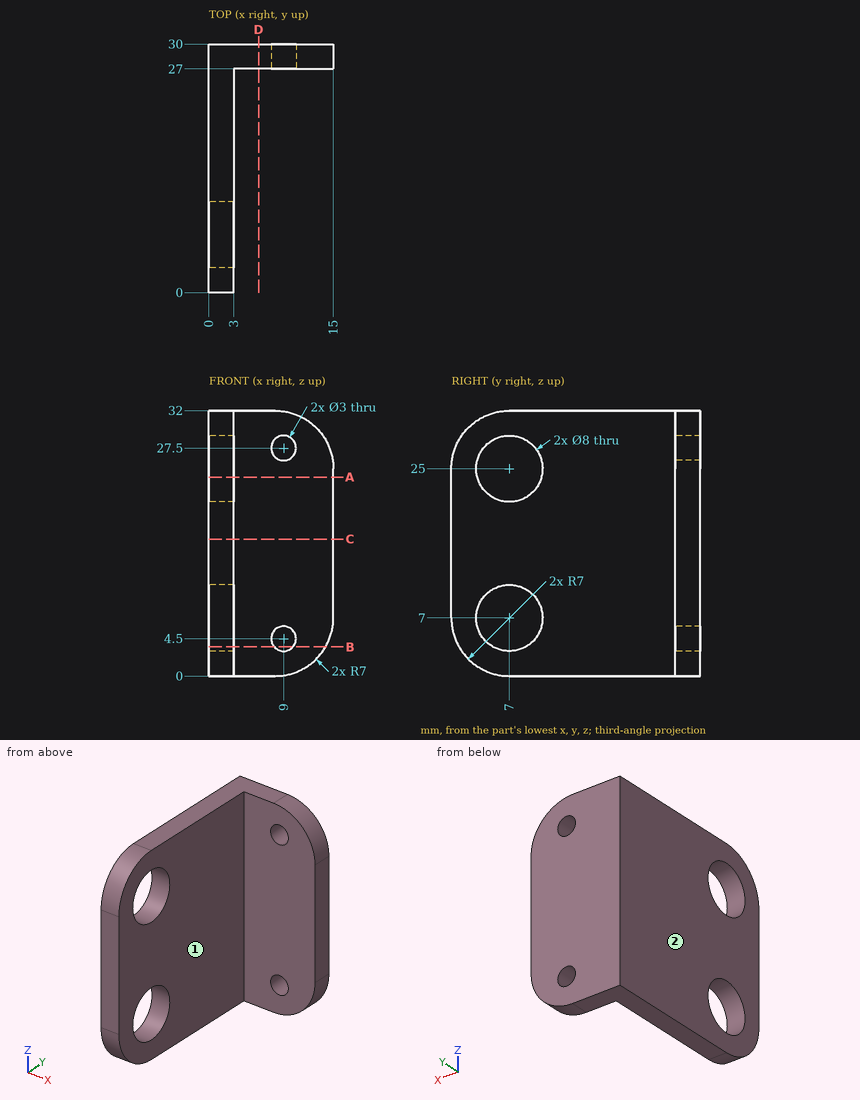
Input: dimensioned drawing with shaded views. Units: mm. Origin: part minimum x, y, z. A direction names the side the tool comes from. Give positions to 0.01 mm unless a question says otherwise; leave off trailing zeros. Loops run counter-clockwise (first coordinate to the right, second up) from the corner with the lowest first, then second, coordinate; pieces in that order, holes last. Notation, with made-up numbers: (16, 76) -> (28, 76) arc R21 cw to (28, 109) -> close; hole circle Ø3 at (-28.5, 77.5). An arc over 180 degrees is marked (long way). Use a Markdown table: item, result. Add a question column.
1) Section query C-C, the plane z = 16.5. Return the cut outline in (x, y), then the cut area to 3 significant figures.
2) Section query A-A, the plane z = 24. Return the cut outline in (x, y), then the cut area to 3 significant figures.
3) Section query B-B, the plane z = 3.5. Return the cut outline in (x, y).
4) Line query: line 1 along Z through (x, y) = (1.1, 7); line 2 along Z through (x, y) = (2.75, 4); line 3 along Y through (x, z) = (1.25, 25). Output: solid intervals per line, ascending. Write a range as [from, to].
5) Section query D-D, the plane x = 6. Return the cut outline in (y, z), then the cut area to 3 significant figures.
6) Reachability of the marked faces 1 and 2 from +Z, -Z, +X, -X, +Y, -Y: full face, straight path, thin tool, end or side. Return the list, or none.
7) First-contact query: pin 1 (5 mm diameter, centred on y = 19.5, z = 27.5, fed in from +X); pin 2 (5 mm diameter, centred on x = 9, z = 4.5, fed in from -Y). Flat tips, straight axial feed; report the tip coordinate or a pass-through.
Numbers:
| question | item | result |
|---|---|---|
| 1 | outline | (0, 0) -> (3, 0) -> (3, 27) -> (15, 27) -> (15, 30) -> (0, 30) -> close |
| 1 | area | 126 mm2 |
| 2 | outline | (0, 0) -> (3, 0) -> (3, 3.13) -> (0, 3.13) -> close; (0, 10.87) -> (3, 10.87) -> (3, 27) -> (15, 27) -> (15, 30) -> (0, 30) -> close |
| 2 | area | 103 mm2 |
| 3 | outline | (0, 0.94) -> (3, 0.94) -> (3, 5.06) -> (0, 5.06) -> close; (0, 8.94) -> (3, 8.94) -> (3, 27) -> (7.88, 27) -> (7.88, 30) -> (0, 30) -> close; (10.12, 27) -> (14.06, 27) -> (14.06, 30) -> (10.12, 30) -> close |
| 4 | line 1 | z = [0, 3], [11, 21], [29, 32] |
| 4 | line 2 | z = [0.68, 4.35], [9.65, 22.35], [27.65, 31.32] |
| 4 | line 3 | y = [0, 3], [11, 30] |
| 5 | outline | (27, 0) -> (30, 0) -> (30, 32) -> (27, 32) -> close |
| 5 | area | 96.0 mm2 |
| 6 | face 1 | +Z, -Z, +X, -Y |
| 6 | face 2 | +Z, -Z, -X, +Y, -Y |
| 7 | pin 1 | stops at x = 3 |
| 7 | pin 2 | stops at y = 27 |
